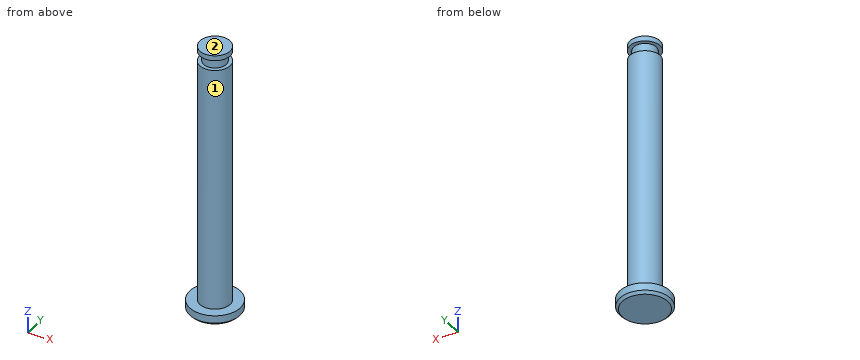
Autodesk Inventor part; units mm, degrees
ref_plane "YZ Plane" through (0, 0, 0) normal (1, 0, 0) x (0, 1, 0)
ref_plane "XZ Plane" through (0, 0, 0) normal (0, 1, 0) x (-1, 0, 0)
ref_plane "XY Plane" through (0, 0, 0) normal (0, 0, 1) x (1, 0, 0)
sketch "スケッチ1" plane through (0, 0, 0) normal (0, 0, 1) x (1, 0, 0)
  circle A0 centre (0, 0) radius 3
  dimension "d0" = 6
extrude "押し出し1" add sketch "スケッチ1" along normal blind 47.8
sketch "スケッチ2" plane through (0, 0, 0) normal (0, 0, -1) x (-1, 0, 0)
  circle A0 centre (0, 0) radius 3
  circle A1 centre (0, 0) radius 5
  dimension "d3" = 10
extrude "押し出し2" add sketch "スケッチ2" along normal blind 2 contours A0 | A1
sketch "スケッチ3" plane through (0, 0, 47.8) normal (0, 0, 1) x (1, 0, 0)
  circle A0 centre (0, 0) radius 3
extrude "押し出し3" add sketch "スケッチ3" along normal blind 1
sketch "スケッチ4" plane through (0, 0, 48.8) normal (0, 0, 1) x (1, 0, 0)
  circle A0 centre (0, 0) radius 3
  circle A1 centre (0, 0) radius 2.25
  dimension "d8" = 4.5
extrude "押し出し4" add sketch "スケッチ4" along normal blind 2 contours A1
sketch "スケッチ5" plane through (0, 0, 50.8) normal (0, 0, 1) x (1, 0, 0)
  circle A0 centre (0, 0) radius 2.25
  circle A1 centre (0, 0) radius 3
  dimension "d11" = 6
extrude "押し出し5" add sketch "スケッチ5" along normal blind 1 contours A0 | A1
chamfer "面取り1" distance 0.5 angle 45 1 edges at (5, 0, -2)
properties part number "shaft6-47.8" material "ステンレス鋼"
Check sheet for the modelled part. Datum: model origin and axes. Units: mm. Face numbers are marked on the shaded views. A direction names the side the tool comes from. Round coordinates to 2 decimals unless told otherwise and drop trailing zeros. Order: outer loops, then holes, each group sorted by start corner. A loop starts at its lowest first (then second) coordinate and runs counter-clockwise, first axis right, second up.
1) Tool access check on the marked faces 1 and 2. Record the directions out of +Z, -Z, +X, -X, +Y, -Y that give a thin tool (end or side, any length) a straight path to the whole face; none if there is none.
2) Go/stop test with flat-tipped pins: pin 1 Ø4 at (x, z) = (1.5, 12) entering from +Y; pin 2 Ø5 at (y, z) = (-2, 44.5) entering from -X; pin 3 Ø6 at (y, z) = (0.5, 45.5) entering from +X. Record where each tip stops, or that it passes through.
3) Scan lines: line 1 (Z direction, x = 0, y = 2.5); line 2 (Z direction, x = -1.25, y = 4); line 3 (Y direction, x = -0.25, z = 9). Record each from-to range of solid material in increasing order.
4) Section check C-C (z = 9). Record the boundary of the cut face in (x, y).
5) Section check A-A (y = 0). Record the boundary of the cut face in (x, z).
Result:
1. face 1: +Z
1. face 2: +Z, +X, -X, +Y, -Y
2. pin 1: stops at y = 3
2. pin 2: stops at x = -3
2. pin 3: stops at x = 3
3. line 1: z = -2 to 48.8, 50.8 to 51.8
3. line 2: z = -2 to 0
3. line 3: y = -2.99 to 2.99
4. outline: circle Ø6 at (0, 0)
5. outline: (-5, -1.5) - (-4.5, -2) - (4.5, -2) - (5, -1.5) - (5, 0) - (3, 0) - (3, 48.8) - (2.25, 48.8) - (2.25, 50.8) - (3, 50.8) - (3, 51.8) - (-3, 51.8) - (-3, 50.8) - (-2.25, 50.8) - (-2.25, 48.8) - (-3, 48.8) - (-3, 0) - (-5, 0) - close
